Source: CAD feature listing. Evaluate the final solid. Frame: model axes, mm. A direction names the side the tool comes from. Coordinates: 2 decimals unless noted, no trailing zeros. Write each loop counter-clockwise with the first axis right and the second up, starting at its lowest first coordinate (ties: lowest second). Pieces come first, ordered by that corner, then holes. Notation, with made-up numbers: M 65,-9.75 L 116,-9.75 A35 cw 116,26.25 Z; hole C 72.25,6 d8. An arc over 180 degrees is marked long. Answer as CSV lines item,"result". Start each with the question number.
1. Section C-C on z = -9. Return the cut outline in (x, y), plus the area to 3 significant figures.
2. Contact query for flat-ended pins moving along their axis: pin 1 Ø12 at (x, z) = (-4.5, -11) entering from +Y; pin 2 Ø4 at (y, z) = (-3.5, -13.5) entering from +X; pin 3 Ø6 at (x, z) = (4, -36) entering from +Y; pin 4 Ø2 at (y, z) = (-8.5, 7) entering from -X. Output: stop coordinate, or through.
3. Line query: probe 1 along Z at (x, y) = (8, -5.5); probe 2 along Y at (x, z) = (0, 0); probe 3 along Y at (x, z) = (3.25, 16.5). Output: solid intervals per line, ascending. Write a range as [from, to].
4. Reachability of faces 1 (the face through (2, 1, -50.896)), 2 (the face through (11.923, -3.755, 43.386)), 3 (the face through (-0.54, -2.44, -35.23)) from +Z, -Z, +X, -X, +Y, -Y: full face, straight path, thin tool, end or side. Return the list, or none.
5. Section D-D on z = -34. Return the cut outline in (x, y), plus the area to 3 significant figures.
6. Mould query, pull axis Z, two halves, no side actions, for faces 4 (the face through (0.37, -1.66, -52.13)), 5 (the face through (-1.46, 6.59, 11.89)), 6 (the face through (5, 5, 42.154)). Classes: pulls with the +Z half, pulls with the -Z half, needs draft (parallel to the pull), parting line crosses it, or undercut.
7. Section A-A on x = 0. Return the cut outline in (y, z), plus the area to 3 significant figures.
```python
from build123d import *

# Parameters (mm, degrees)
ESBO_O2_R                = 12.5
ESBO_O2_R_2              = 6.75
CORTE_EXTRUS_O1_DEPTH    = 1.5
ESBO_O3_R                = 2.5
RESSALTO_EXTRUS_O1_DEPTH = 104.8
CORTE_EXTRUS_O2_START    = -2.5
ESBO_O4_R                = 2.5
ESBO_O4_R_2              = 1.7
CORTE_EXTRUS_O2_DEPTH    = 2.5


with BuildPart() as part:
    # Esboço1 → Revolução1 (revolve)
    with BuildSketch(Plane(origin=(0, 0, 0), x_dir=(0, 0, -1), z_dir=(1, 0, 0)), mode=Mode.PRIVATE) as revolu_o1_sk:
        Polygon((-44.653738644, 0), (-44.653738644, -12.5), (-40.653738644, -12.5), (-40.653738644, -6.75), (17.546261356, -6.75), (20, -2.5), (0, -2.5), (0, 0), align=None)
    revolve(revolu_o1_sk.sketch.rotate(Axis((0, 0, 72.391069924), (0, 0, -1)), 270), axis=Axis((0, 0, 72.391069924), (0, 0, -1)))

    # Esboço2 → Corte-extrusão1 (cut)
    with BuildSketch(Plane(origin=(0, 0, 40.653738644), x_dir=(-1, 0, 0), z_dir=(0, 0, -1))):
        with Locations(Location((0, 0, 0), (0, 0, 180))):
            Circle(ESBO_O2_R)
        with Locations(Location((0, 0, 0), (0, 0, 180))):
            Circle(ESBO_O2_R_2, mode=Mode.SUBTRACT)
    extrude(amount=-CORTE_EXTRUS_O1_DEPTH, mode=Mode.SUBTRACT)

    # Esboço3 → Ressalto-extrusão1 (add)
    with BuildSketch(Plane.XY.offset(44.653738644)):
        Circle(ESBO_O3_R)
    extrude(amount=-RESSALTO_EXTRUS_O1_DEPTH)

    # Esboço4 → Corte-extrusão2 (cut)
    with BuildSketch(Plane(origin=(0, 0, -53.396261356), x_dir=(-1, 0, 0), z_dir=(0, 0, -1)).offset(CORTE_EXTRUS_O2_START)):
        with Locations(Location((0, 0, 0), (0, 0, 180))):
            Circle(ESBO_O4_R)
        Circle(ESBO_O4_R_2, mode=Mode.SUBTRACT)
    extrude(amount=CORTE_EXTRUS_O2_DEPTH, mode=Mode.SUBTRACT)


solid = part.part
```
Values:
1,outline,"C 0,0 d13.5"
1,area,"143 mm²"
2,pin 1,"y = 6.75"
2,pin 2,"x = 6.58"
2,pin 3,"y = 2.29"
2,pin 4,"through"
3,probe 1,"[42.15, 44.65]"
3,probe 2,"[-6.75, 6.75]"
3,probe 3,"[-5.92, 5.92]"
4,face 1,"none"
4,face 2,"+Z, -Z"
4,face 3,"-Z"
5,outline,"C 0,0 d5"
5,area,"19.6 mm²"
6,face 4,"undercut"
6,face 5,"needs draft"
6,face 6,"pulls with the -Z half"
7,outline,"M -12.5,42.15 L -6.75,42.15 L -6.75,-17.55 L -2.5,-20 L -2.5,-50.9 L -1.7,-50.9 L -1.7,-53.4 L -2.5,-53.4 L -2.5,-60.15 L 2.5,-60.15 L 2.5,-53.4 L 1.7,-53.4 L 1.7,-50.9 L 2.5,-50.9 L 2.5,-20 L 6.75,-17.55 L 6.75,42.15 L 12.5,42.15 L 12.5,44.65 L -12.5,44.65 Z"
7,area,"1,090 mm²"
